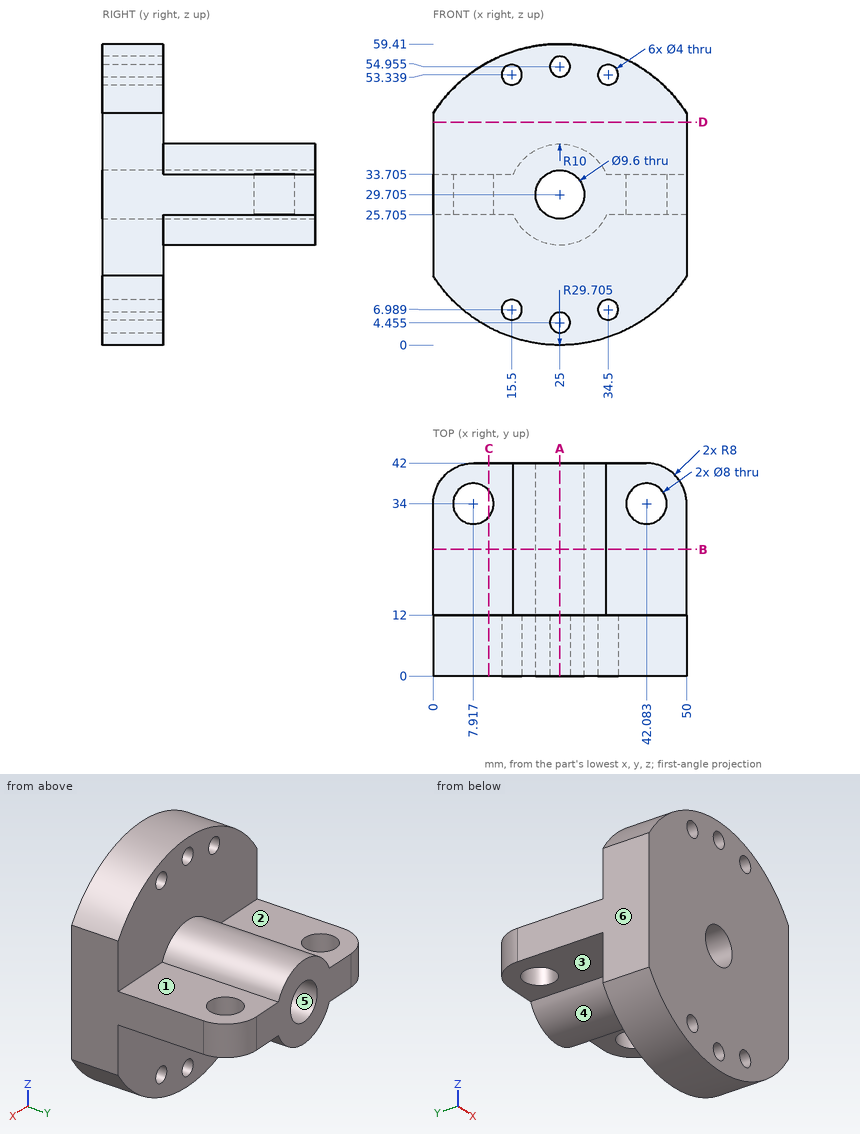
Source: three-view drawing plus pictorial views. Frame: mm from the lowest corner of the part. A direction names the side the tool comes from. Round coordinates to 2 decimals unless told otherwise and drop trailing zeros. Order: outer loops, then holes, each group sorted by start corner. A loop starts at its lowest first (then second) coordinate and runs counter-clockwise, first axis right, second up. Notation, with made-up numbers: (20, 72) -> (26, 72) arc R25 ccw to (26, 91) -> close; hole circle Ø3 at (-5, -22). An arc over 180 degrees is marked (long way). Use one line per item in the form item = value.
(1) Access query for the marked faces 1, 2 and 3. Directions: +Z, -Z, +X, -X, +Y, -Y. A direction counts if a zero-diameter tool reaches every point of the face in a straight line with its end or side. Return the directions, or none.
Results list:
face_1 = +Z, +X, +Y
face_2 = +Z, -X, +Y
face_3 = -Z, -X, +Y
(2) Section C-C on x = 11. Return loops of the section in (y, z) (1 decimal).
Results list:
outline = (0, 3.5) -> (12, 3.5) -> (12, 25.7) -> (31.5, 25.7) -> (31.5, 33.7) -> (12, 33.7) -> (12, 55.9) -> (0, 55.9) -> close; (36.5, 25.7) -> (42, 25.7) -> (42, 33.7) -> (36.5, 33.7) -> close
(3) Ray query, probe 1 along X at (y, z) = (28, 29.5) (1 decimal); probe 2 along Z at (x, y) = (34, 3) (1 decimal); probe 3 along Y at (x, z) = (7, 36). Return the intervals inside material, ascending. Write a range as [from, to].
Results list:
probe_1 = [0, 20.2], [29.8, 50]
probe_2 = [1.4, 5.1], [8.9, 51.4], [55.3, 58]
probe_3 = [0, 12]
(4) First-contact query: pin 1 Ø4.5 at (x, z) = (34.5, 6.99) entering from +Y; pin 2 Ø5 at (x, y) = (37, 24.5) entering from -Z (3 decimals); pin 3 Ø12 at (x, y) = (21.5, 24.5) entering from +Z (3 decimals). Flat tips, straight axial feed; report the tip coordinate or a pass-through.
Results list:
pin_1 = 12
pin_2 = 25.705
pin_3 = 39.705
(5) Section D-D on z = 44. Return loops of the section in (x, y), and give its area (3 significant figures).
Results list:
outline = (0, 0) -> (50, 0) -> (50, 12) -> (0, 12) -> close
area = 600 mm^2
(6) Section B-B on y = 25. Return loops of the section in (x, z) (1 decimal), and give its area (3 significant figures).
Results list:
outline = (0, 25.7) -> (15.8, 25.7) arc R10 ccw to (34.2, 25.7) -> (50, 25.7) -> (50, 33.7) -> (34.2, 33.7) arc R10 ccw to (15.8, 33.7) -> (0, 33.7) -> close; hole circle Ø9.6 at (25, 29.7)
area = 486 mm^2
(7) Section A-A on x = 25. Return loops of the section in (y, z) (1 decimal).
Results list:
outline = (0, 0) -> (12, 0) -> (12, 2.5) -> (0, 2.5) -> close; (0, 6.5) -> (12, 6.5) -> (12, 19.7) -> (42, 19.7) -> (42, 24.9) -> (0, 24.9) -> close; (0, 34.5) -> (42, 34.5) -> (42, 39.7) -> (12, 39.7) -> (12, 53) -> (0, 53) -> close; (0, 57) -> (12, 57) -> (12, 59.4) -> (0, 59.4) -> close
(8) Draft query along X for the marked faces 4, 5 and 6. Return one class per face: pulls with the +X half, pulls with the -X half, needs draft (parallel to the pull), parting line crosses it, or undercut.
Results list:
face_4 = parting line crosses it
face_5 = undercut
face_6 = pulls with the -X half
